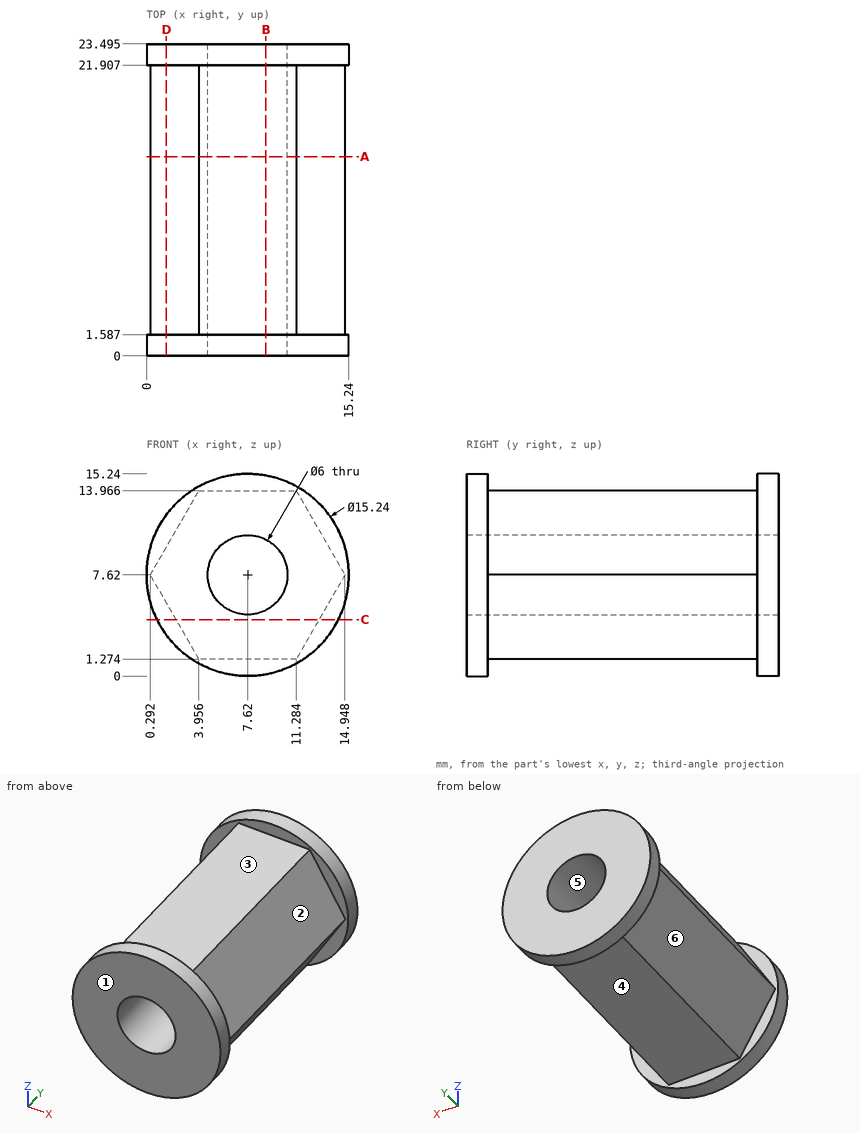
Design review of the part shown in the three views and the two pictorial views. Dimensions are in mm from the part's minimum x, y and z. A direction names the side the tool comes from. Round coordinates to 2 decimals unless told otherwise and drop trailing zeros. Loops run counter-clockwise (first coordinate to the right, second up) from the corner with the lowest first, then second, coordinate; pieces in that order, holes last. Notation, with made-up numbers: (-30.5, 3.25) -> (4.5, 3.25) arc R23 ccw to (4.5, 31.25) -> close; hole circle Ø9 at (37.25, 19). An arc over 180 degrees is marked (long way). Answer as CSV lines item,"result".
1) Tool access review of the marked faces 1, 2 and 3: name each direction out of +Z, -Z, +X, -X, +Y, -Y from which nothing blocks a thin tool from reaching the whole face with its end or side.
Geometry results:
face 1,"+Z, -Z, +X, -X, -Y"
face 2,"+Z, +X"
face 3,"+Z, +X, -X"
2) Add section D-D on x = 1.5. Write out the cut boundary in (y, z) (1 decimal), plus the area to 3 significant figures.
Geometry results:
outline,"(0, 3.1) -> (1.6, 3.1) -> (1.6, 5.5) -> (21.9, 5.5) -> (21.9, 3.1) -> (23.5, 3.1) -> (23.5, 12.2) -> (21.9, 12.2) -> (21.9, 9.7) -> (1.6, 9.7) -> (1.6, 12.2) -> (0, 12.2) -> close"
area,"114 mm²"
3) Add section C-C on z = 4.25. Write out the cut boundary in (x, y) (1 decimal), plus the area to 3 significant figures.
Geometry results:
outline,"(0.8, 0) -> (14.5, 0) -> (14.5, 1.6) -> (13, 1.6) -> (13, 21.9) -> (14.5, 21.9) -> (14.5, 23.5) -> (0.8, 23.5) -> (0.8, 21.9) -> (2.2, 21.9) -> (2.2, 1.6) -> (0.8, 1.6) -> close"
area,"262 mm²"
4) For P1, Ø6, axis at x = 7, y = 7, coming from the +Z side; P2, Ø8, axis at x = 3.5, y = 20, coming from the +Z side; P3, Ø5, axis at x = 12.5, y = 6, coming from the -Z side, all flat-tipped, find the tip position at first contact; note any pin that passes through.
Geometry results:
P1,"stops at z = 13.97"
P2,"stops at z = 15.22"
P3,"stops at z = 1.27"
5) To check wall thickness, follow line 1 along Y through (x, z) = (14.75, 9.75) (1 decimal); line 2 along X through (y, z) = (6.5, 5.75) (1 decimal); line 3 along Z through (x, y) = (9.75, 3.25) (1 decimal). State the ranges of each line that lie inside material, in increasing order. Write a range as from..to.
Geometry results:
line 1,"y = 0..1.6, 21.9..23.5"
line 2,"x = 1.4..5.3, 10..13.9"
line 3,"z = 1.3..5.5, 9.7..14"
6) Draft analysis for pull direction X (two halves, no side actions). For the marked faces 4, 5 and 6, state which applies: pulls with the +X half, pulls with the -X half, needs draft (parallel to the pull), parting line crosses it, or undercut.
Geometry results:
face 4,"needs draft"
face 5,"undercut"
face 6,"pulls with the -X half"
7) Add section A-A on y = 15. Write out the cut boundary in (x, z).
Geometry results:
outline,"(0.29, 7.62) -> (3.96, 1.27) -> (11.28, 1.27) -> (14.95, 7.62) -> (11.28, 13.97) -> (3.96, 13.97) -> close; hole circle Ø6 at (7.62, 7.62)"
8) Add section B-B on x = 9. Write out the cut boundary in (y, z) (1 decimal).
Geometry results:
outline,"(0, 0.1) -> (1.6, 0.1) -> (1.6, 1.3) -> (21.9, 1.3) -> (21.9, 0.1) -> (23.5, 0.1) -> (23.5, 5) -> (0, 5) -> close; (0, 10.3) -> (23.5, 10.3) -> (23.5, 15.1) -> (21.9, 15.1) -> (21.9, 14) -> (1.6, 14) -> (1.6, 15.1) -> (0, 15.1) -> close"
